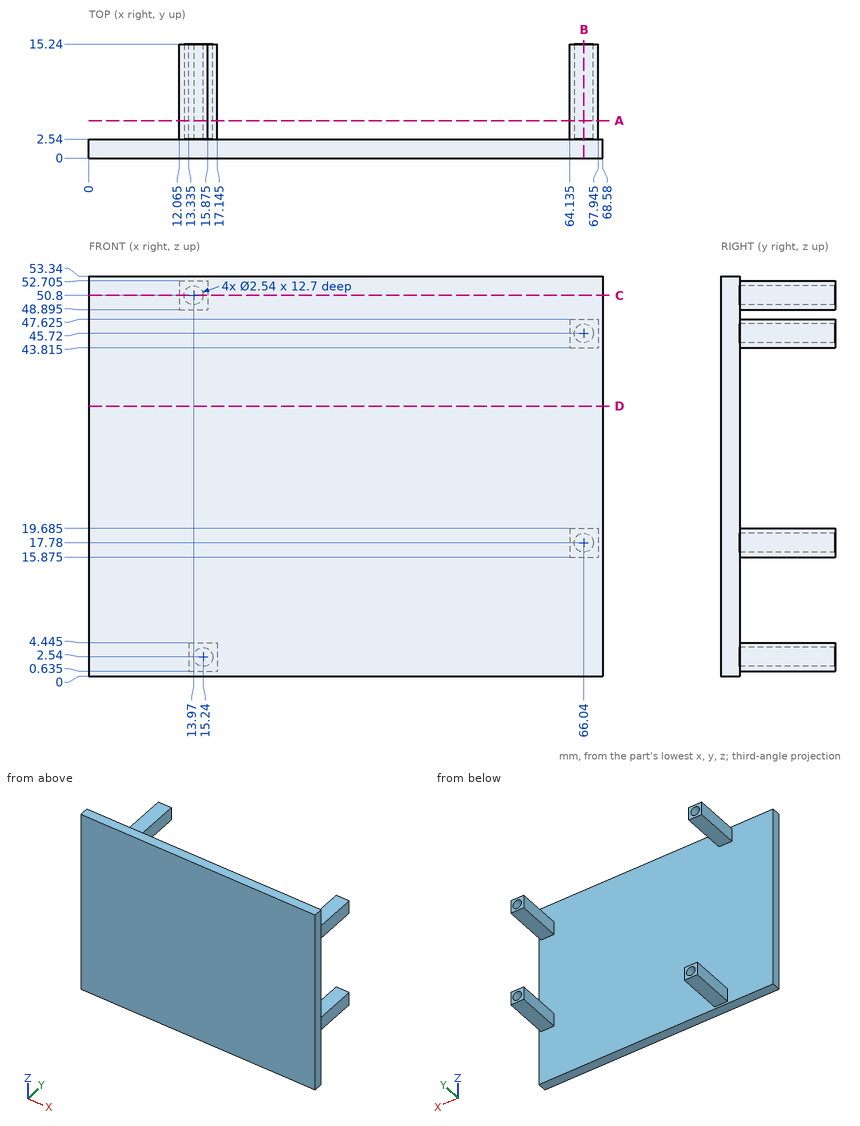
Check sheet for the drawn part. Datum: minimum x, y, z corner. Units: mm. Round coordinates to 2 decimals unless told otherwise and drop trailing zeros. Loops run counter-clockwise (first coordinate to the right, second up) from the corner with the lowest first, then second, coordinate; pieces in that order, holes last. Notation, with made-up numbers: M 46.25,-31.5 L 98.25,-31.5 A30 cw 98.25,-9.5 Z; hole C 26,55.5 d5. An arc over 180 degrees is marked long. One line per question, with ' | ' between items. Start each with the question number.
Item 1: Section check B-B (x = 66.04). Record the boundary of the cut face in (y, z) (3 decimals), and give its area (3 significant figures).
Item 2: Section check D-D (z = 36). Record the boundary of the cut face in (x, y), and give its area (3 significant figures).
Item 3: Scan lines: probe 1 along X at (y, z) = (4, 44) (3 decimals); probe 2 along Y at (x, z) = (49, 19.5); probe 3 along Z at (x, y) = (17, 12) (3 decimals). Record each from-to range of solid material in increasing order.
Item 4: Section check C-C (z = 50.8). Record the boundary of the cut face in (x, y) (3 decimals).
Item 5: Gauge pin test, flat ends, axial feed: pin 1 Ø1.1 at (x, y) = (67, 9.5) entering from -Z (3 decimals); pin 2 Ø1.9 at (x, y) = (65.5, 9.5) entering from +Z (3 decimals); pin 3 Ø3 at (y, z) = (10.5, 2) entering from +X (3 decimals). Record the tip position at first contact, or that the pin passes through.
Item 6: Section check A-A (y = 5). Record the boundary of the cut face in (x, z) (3 decimals), and give its area (3 significant figures).
Worked out:
1) outline: M 0,0 L 2.54,0 L 2.54,15.875 L 15.24,15.875 L 15.24,16.51 L 2.54,16.51 L 2.54,19.05 L 15.24,19.05 L 15.24,19.685 L 2.54,19.685 L 2.54,43.815 L 15.24,43.815 L 15.24,44.45 L 2.54,44.45 L 2.54,46.99 L 15.24,46.99 L 15.24,47.625 L 2.54,47.625 L 2.54,53.34 L 0,53.34 Z | area: 168 mm^2
2) outline: M 0,0 L 68.58,0 L 68.58,2.54 L 0,2.54 Z | area: 174 mm^2
3) probe 1: 64.135 to 67.945 | probe 2: 0 to 2.54 | probe 3: 0.635 to 4.445
4) outline: M 0,0 L 68.58,0 L 68.58,2.54 L 15.875,2.54 L 15.875,15.24 L 15.24,15.24 L 15.24,2.54 L 12.7,2.54 L 12.7,15.24 L 12.065,15.24 L 12.065,2.54 L 0,2.54 Z
5) pin 1: z = 15.875 | pin 2: z = 47.625 | pin 3: x = 17.145
6) outline: M 12.065,48.895 L 15.875,48.895 L 15.875,52.705 L 12.065,52.705 Z; M 13.335,0.635 L 17.145,0.635 L 17.145,4.445 L 13.335,4.445 Z; M 64.135,15.875 L 67.945,15.875 L 67.945,19.685 L 64.135,19.685 Z; M 64.135,43.815 L 67.945,43.815 L 67.945,47.625 L 64.135,47.625 Z; hole C 13.97,50.8 d2.54; hole C 15.24,2.54 d2.54; hole C 66.04,17.78 d2.54; hole C 66.04,45.72 d2.54 | area: 37.8 mm^2
